from build123d import *

# Parameters (mm, degrees)
BOSS_EXTRUDE1_DEPTH = 558.8
SKETCH2_R           = 2.667
CUT_EXTRUDE1_DEPTH  = 564.121852377
SKETCH3_R           = 2.667
CUT_EXTRUDE2_DEPTH  = 564.121852377


with BuildPart() as part:
    # Sketch1 → Boss-Extrude1 (new body)
    with BuildSketch(Plane.XY):
        with BuildLine():
            Line((3.175, 50.8), (3.175, 3.937))
            ThreePointArc((3.175, 3.937), (3.398184633, 3.398184633), (3.937, 3.175))
            Line((3.937, 3.175), (50.8, 3.175))
            Line((50.8, 3.175), (50.8, 0))
            Line((50.8, 0), (0.762, 0))
            ThreePointArc((0.762, 0), (0.223184633, 0.223184633), (0, 0.762))
            Line((0, 0.762), (0, 50.8))
            Line((0, 50.8), (3.175, 50.8))
        make_face()
    extrude(amount=BOSS_EXTRUDE1_DEPTH)

    # Sketch2 → Cut-Extrude1 (cut, through all)
    with BuildSketch(Plane(origin=(0, 3.175, 0), x_dir=(1, 0, 0), z_dir=(0, 1, 0))):
        with Locations(Location((34.163, -6.35, 0), (0, 0, 270))):
            Circle(SKETCH2_R)
        with Locations(Location((8.763, -6.35, 0), (0, 0, 270))):
            Circle(SKETCH2_R)
    extrude(amount=-CUT_EXTRUDE1_DEPTH, mode=Mode.SUBTRACT)

    # Sketch3 → Cut-Extrude2 (cut, through all)
    with BuildSketch(Plane(origin=(3.175, 0, 0), x_dir=(0, 0, -1), z_dir=(1, 0, 0))):
        with Locations(Location((-552.45, 34.163, 0), (0, 0, 90))):
            Circle(SKETCH3_R)
        with Locations(Location((-552.45, 8.763, 0), (0, 0, 90))):
            Circle(SKETCH3_R)
    extrude(amount=-CUT_EXTRUDE2_DEPTH, mode=Mode.SUBTRACT)


solid = part.part
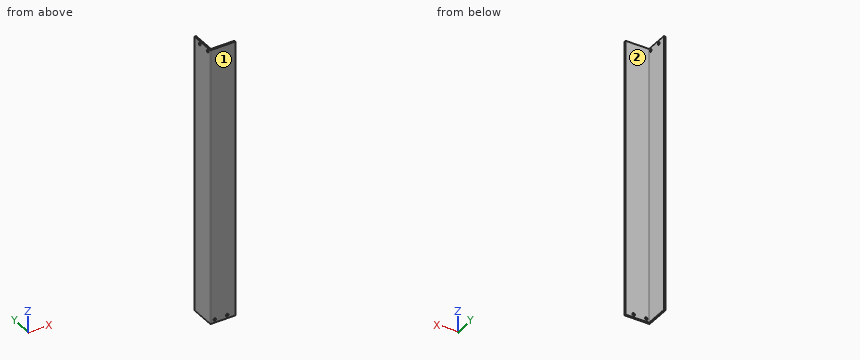
Source: CAD feature listing. Evaluate the final solid. Frame: model axes, mm. Face numbers are marked on the shaded views. A direction names the side the tool comes from. Coordinates: 2 decimals unless noted, no trailing zeros. Order: outer loops, then holes, each group sorted by start corner. A loop starts at its lowest first (then second) coordinate and runs counter-clockwise, first axis right, second up. Notation, with made-up numbers: M 86,54 L 107,54 A10 cw 107,68 Z; hole C 66,-9.75 d6. An arc over 180 degrees is marked long. Write each question's results on one line, items separated by ' | '. Start each with the question number.
Item 1: Cut plane B-B (y = 22). Return loops of the section in (x, z) (3 decimals).
Item 2: Cut plane A-A (z = 188). Return loops of the section in (x, y) (3 decimals).
Item 3: First-contact query: pin 1 Ø4.5 at (y, z) = (8.763, 552.45) entering from +X (3 decimals); pin 2 Ø6 at (x, z) = (34.163, 6.35) entering from +Y (3 decimals); pin 3 Ø10 at (y, z) = (32, 181) entering from +X (3 decimals). Flat tips, straight axial feed; report the tip coordinate or a pass-through.
Item 4: Set-up query: the marked faces 1 and 2. Return all of +Z, -Z, +X, -X, +Y, -Y with unobstructed straight access to the full face (end or side cutting, diameter ignored); none if empty.
Item 5: Line query: probe 1 along X at (y, z) = (1.15, 6.35); probe 2 along Y at (x, z) = (26, 262) (3 decimals). Output: solid intervals per line, ascending.
Checked values:
1) outline: M 0,0 L 3.175,0 L 3.175,558.8 L 0,558.8 Z
2) outline: M 0,0.762 A0.762 ccw 0.762,0 L 50.8,0 L 50.8,3.175 L 3.937,3.175 A0.762 cw 3.175,3.937 L 3.175,50.8 L 0,50.8 Z
3) pin 1: passes through | pin 2: stops at y = 3.175 | pin 3: stops at x = 3.175
4) face 1: +Z, -Z, +X, -X, -Y | face 2: +Z, -Z, +X, +Y
5) probe 1: x = 0 to 6.1, 11.43 to 31.5, 36.83 to 50.8 | probe 2: y = 0 to 3.175
